Autodesk Inventor part; units mm, degrees
ref_plane "YZ Plane" through (0, 0, 0) normal (1, 0, 0) x (0, 1, 0)
ref_plane "XZ Plane" through (0, 0, 0) normal (0, 1, 0) x (-1, 0, 0)
ref_plane "XY Plane" through (0, 0, 0) normal (0, 0, 1) x (1, 0, 0)
sketch "Skizze1" plane through (0, 0, 0) normal (0, 0, 1) x (1, 0, 0)
  circle A0 centre (-60.768, 178.1277) radius 7
  circle A1 centre (-40.718, 169.3777) radius 1.6
  circle A2 centre (-40.718, 186.8777) radius 1.6
  line L0 (-23.718, 156.1277) -> (-23.718, 166.1277)
  arc A3 (-23.718, 166.1277) -> (-28.718, 171.1277) centre (-28.718, 166.1277) ccw
  line L1 (-28.718, 171.1277) -> (-29.418, 171.1277)
  arc A4 (-29.418, 185.1277) -> (-29.418, 171.1277) centre (-29.418, 178.1277) ccw
  line L2 (-40.918, 197.1277) -> (-40.918, 200.6277)
  line L3 (-40.918, 200.6277) -> (-60.918, 200.6277)
  line L4 (-68.918, 197.1277) -> (-76.918, 197.1277)
  line L5 (-76.918, 197.1277) -> (-76.918, 159.1277)
  line L6 (-76.918, 159.1277) -> (-68.918, 159.1277)
  line L7 (-64.918, 159.1277) -> (-26.718, 159.1277)
  line L8 (-26.718, 159.1277) -> (-26.718, 156.1277)
  line L9 (-26.718, 156.1277) -> (-23.718, 156.1277)
  line L10 (-36.5327, 178.1277) -> (-67.768, 178.1277) construction
  line L11 (-40.718, 169.3777) -> (-40.718, 186.8777) construction
  line L12 (-32.918, 197.1277) -> (-32.918, 193.6277)
  line L13 (-32.918, 193.6277) -> (-31.418, 193.6277)
  line L14 (-31.418, 193.6277) -> (-31.418, 190.1277)
  line L15 (-31.418, 190.1277) -> (-32.918, 190.1277)
  line L16 (-32.918, 190.1277) -> (-32.918, 188.6277)
  line L17 (-32.918, 188.6277) -> (-36.918, 188.6277)
  line L18 (-36.918, 188.6277) -> (-36.918, 190.1277)
  line L19 (-36.918, 190.1277) -> (-38.418, 190.1277)
  line L20 (-38.418, 190.1277) -> (-38.418, 193.6277)
  line L21 (-38.418, 193.6277) -> (-36.918, 193.6277)
  line L22 (-36.918, 197.1277) -> (-36.918, 193.6277)
  line L23 (-34.918, 197.9429) -> (-34.918, 190.1833) construction
  line L24 (-32.918, 197.1277) -> (-24.918, 197.1277)
  line L25 (-50.918, 190.3199) -> (-50.918, 199.5586) construction
  line L26 (-68.918, 190.1277) -> (-68.918, 188.6277)
  line L27 (-66.918, 197.9429) -> (-66.918, 190.1833) construction
  line L28 (-64.918, 197.1277) -> (-64.918, 193.6277)
  line L29 (-68.918, 188.6277) -> (-64.918, 188.6277)
  line L30 (-63.418, 193.6277) -> (-64.918, 193.6277)
  line L31 (-63.418, 190.1277) -> (-63.418, 193.6277)
  line L32 (-64.918, 188.6277) -> (-64.918, 190.1277)
  line L33 (-64.918, 190.1277) -> (-63.418, 190.1277)
  line L34 (-70.418, 190.1277) -> (-68.918, 190.1277)
  line L35 (-68.918, 193.6277) -> (-70.418, 193.6277)
  line L36 (-70.418, 193.6277) -> (-70.418, 190.1277)
  line L37 (-68.918, 197.1277) -> (-68.918, 193.6277)
  line L38 (-29.418, 185.1277) -> (-24.918, 185.1277)
  line L39 (-24.918, 185.1277) -> (-24.918, 197.1277)
  line L40 (-60.918, 200.6277) -> (-60.918, 197.1277)
  line L41 (-36.918, 197.1277) -> (-40.918, 197.1277)
  line L42 (-60.918, 197.1277) -> (-64.918, 197.1277)
  line L43 (-68.918, 162.6277) -> (-70.418, 162.6277)
  line L44 (-70.418, 162.6277) -> (-70.418, 166.1277)
  line L45 (-70.418, 166.1277) -> (-68.918, 166.1277)
  line L46 (-68.918, 166.1277) -> (-68.918, 167.6277)
  line L47 (-68.918, 167.6277) -> (-64.918, 167.6277)
  line L48 (-64.918, 167.6277) -> (-64.918, 166.1277)
  line L49 (-64.918, 166.1277) -> (-63.418, 166.1277)
  line L50 (-63.418, 166.1277) -> (-63.418, 162.6277)
  line L51 (-63.418, 162.6277) -> (-64.918, 162.6277)
  line L52 (-64.918, 159.1277) -> (-64.918, 162.6277)
  line L53 (-68.918, 159.1277) -> (-68.918, 162.6277)
  circle A5 centre (-49.518, 178.1277) radius 1.95
  point P0 (0, 0)
  point P1 (-56.218, 159.1277)
  point P2 (-36.918, 159.1277)
  point P3 (-40.718, 178.1277)
  dimension "d51" = 14
  dimension "d4" = 14
  dimension "d5" = 3
  dimension "d7" = 5
  dimension "d8" = 7
  dimension "d9" = 4.3
  dimension "d27" = 32
  dimension "d28" = 10
  dimension "d31" = 10
  dimension "d33" = 20
  dimension "d34" = 3.5
  dimension "d37" = 4
  dimension "d38" = 7
  dimension "d39" = 3.5
  dimension "d40" = 3.5
  dimension "d41" = 1.5
  dimension "d42" = 5.8
  dimension "d43" = 22.5
  dimension "d45" = 3
  dimension "d49" = 11.25
  dimension "d50" = 3.9
extrude "Extrusion1" add sketch "Skizze1" along normal mid plane 4 contours L9 L8 L7 L52 L51 L50 L49 L48 L47 L46 L45 L44 L43 L53 L6 L5 L4 L37 L35 L36 L34 L26 L29 L32 L33 L31 L30 L28 L42 L40 L3 L2 L41 L22 L21 L20 L19 L18 L17 L16 L15 L14 L13 L12 L24 L39 L38 A4 L1 A3 L0 | A5
sketch "Skizze2" plane through (0, 0, -2) normal (0, 0, -1) x (-1, 0, 0)
  circle A0 centre (60.768, 178.1277) radius 7
  circle A1 centre (40.718, 186.8777) radius 1.6
  circle A2 centre (40.718, 169.3777) radius 1.6
  line L0 (23.718, 166.1277) -> (23.718, 156.1277)
  line L1 (23.718, 156.1277) -> (26.718, 156.1277)
  line L2 (26.718, 156.1277) -> (26.718, 159.1277)
  line L3 (26.718, 159.1277) -> (64.918, 159.1277)
  line L4 (64.918, 159.1277) -> (64.918, 162.6277)
  line L5 (64.918, 162.6277) -> (63.418, 162.6277)
  line L6 (63.418, 162.6277) -> (63.418, 166.1277)
  line L7 (63.418, 166.1277) -> (64.918, 166.1277)
  line L8 (64.918, 166.1277) -> (64.918, 167.6277)
  line L9 (64.918, 167.6277) -> (68.918, 167.6277)
  line L10 (68.918, 167.6277) -> (68.918, 166.1277)
  line L11 (68.918, 166.1277) -> (70.418, 166.1277)
  line L12 (70.418, 166.1277) -> (70.418, 162.6277)
  line L13 (70.418, 162.6277) -> (68.918, 162.6277)
  line L14 (68.918, 162.6277) -> (68.918, 159.1277)
  line L15 (68.918, 159.1277) -> (76.918, 159.1277)
  line L16 (76.918, 159.1277) -> (76.918, 197.1277)
  line L17 (76.918, 197.1277) -> (68.918, 197.1277)
  line L18 (68.918, 197.1277) -> (68.918, 193.6277)
  line L19 (68.918, 193.6277) -> (70.418, 193.6277)
  line L20 (70.418, 193.6277) -> (70.418, 190.1277)
  line L21 (70.418, 190.1277) -> (68.918, 190.1277)
  line L22 (68.918, 190.1277) -> (68.918, 188.6277)
  line L23 (68.918, 188.6277) -> (64.918, 188.6277)
  line L24 (64.918, 188.6277) -> (64.918, 190.1277)
  line L25 (64.918, 190.1277) -> (63.418, 190.1277)
  line L26 (63.418, 190.1277) -> (63.418, 193.6277)
  line L27 (63.418, 193.6277) -> (64.918, 193.6277)
  line L28 (64.918, 193.6277) -> (64.918, 197.1277)
  line L29 (64.918, 197.1277) -> (60.918, 197.1277)
  line L30 (60.918, 197.1277) -> (60.918, 200.6277)
  line L31 (60.918, 200.6277) -> (40.918, 200.6277)
  line L32 (40.918, 200.6277) -> (40.918, 197.1277)
  line L33 (40.918, 197.1277) -> (36.918, 197.1277)
  line L34 (36.918, 197.1277) -> (36.918, 193.6277)
  line L35 (36.918, 193.6277) -> (38.418, 193.6277)
  line L36 (38.418, 193.6277) -> (38.418, 190.1277)
  line L37 (38.418, 190.1277) -> (36.918, 190.1277)
  line L38 (36.918, 190.1277) -> (36.918, 188.6277)
  line L39 (36.918, 188.6277) -> (32.918, 188.6277)
  line L40 (32.918, 188.6277) -> (32.918, 190.1277)
  line L41 (32.918, 190.1277) -> (31.418, 190.1277)
  line L42 (31.418, 190.1277) -> (31.418, 193.6277)
  line L43 (31.418, 193.6277) -> (32.918, 193.6277)
  line L44 (32.918, 193.6277) -> (32.918, 197.1277)
  line L45 (32.918, 197.1277) -> (24.918, 197.1277)
  line L46 (24.918, 197.1277) -> (24.918, 185.1277)
  line L47 (24.918, 185.1277) -> (29.418, 185.1277)
  arc A3 (29.418, 171.1277) -> (29.418, 185.1277) centre (29.418, 178.1277) ccw
  line L48 (29.418, 171.1277) -> (28.718, 171.1277)
  arc A4 (28.718, 171.1277) -> (23.718, 166.1277) centre (28.718, 166.1277) ccw
  circle A5 centre (40.718, 169.3777) radius 1.6
  line L49 (42.9634, 171.623) -> (43.7853, 168.5558)
  line L50 (43.7853, 168.5558) -> (41.5399, 166.3104)
  line L51 (41.5399, 166.3104) -> (38.4727, 167.1323)
  line L52 (38.4727, 167.1323) -> (37.6508, 170.1995)
  line L53 (37.6508, 170.1995) -> (39.8962, 172.4449)
  line L54 (39.8962, 172.4449) -> (42.9634, 171.623)
  line L55 (42.9634, 189.123) -> (43.7853, 186.0558)
  line L56 (43.7853, 186.0558) -> (41.5399, 183.8104)
  line L57 (41.5399, 183.8104) -> (38.4727, 184.6323)
  line L58 (38.4727, 184.6323) -> (37.6508, 187.6995)
  line L59 (37.6508, 187.6995) -> (39.8962, 189.9449)
  line L60 (39.8962, 189.9449) -> (42.9634, 189.123)
  line L61 (38.418, 190.1277) -> (36.918, 188.6277) construction
  point P0 (0, 0)
  dimension "d52" = 5.5
extrude "Extrusion2" cut sketch "Skizze2" against normal blind 2 contours L49 L50 L51 L52 L53 L54 | L55 L56 L57 L58 L59 L60
sketch "Skizze3" plane through (-64.918, 159.1277, 2) normal (0, -1, 0) x (1, 0, 0)
  line L0 (0, 0) -> (38.2, 0)
  line L1 (12, -4) -> (16, -4)
  line L2 (16, -4) -> (16, 0)
  line L3 (16, 0) -> (12, 0)
  line L4 (12, 0) -> (12, -4)
  line L5 (-12, -4) -> (-12, 0)
  point P0 (64.918, -2)
  point P1 (-2, -2)
  dimension "d55" = 4
  dimension "d57" = 24
extrude "Extrusion3" add sketch "Skizze3" along normal blind 2
properties part number "Motorhalter_links"
Build history of the part. All positions in model axes, mm. A direction names the side the tool comes from. Round coordinates to 2 decimals unless told otherwise and drop trailing zeros. Write each loop counter-clockwise with the first axis right and the second up, starting at its lowest first coordinate (ties: lowest second). Pieces come first, ordered by that corner, then holes. Notation, with made-up numbers: (25, 80) - (45, 80) arc R23 cw to (45, 106) - close; hole circle Ø11 at (69.25, -28.75). An arc over 180 degrees is marked (long way). One line per question, with ' | ' between items.
1. Mould opens along X. For faces 6 (the face through (-60.918, 199, 0)), 7 (the face through (-51, 179, -2)), 8 (the face through (-70.418, 192, 0)) say: released by +X, released by -X, zero draft, split by the parting line, or undercut.
Results are:
face 6: released by -X | face 7: zero draft | face 8: undercut
2. Band-saw the part on B-B, the plane y = 161.5. Write the cut outline in (x, z).
Results are:
outline: (-76.92, -2) - (-68.92, -2) - (-68.92, 2) - (-76.92, 2) - close; (-64.92, -2) - (-23.72, -2) - (-23.72, 2) - (-64.92, 2) - close
3. Band-saw the part on C-C, the plane x = -60. Write the cut outline in (y, z), and give its area (3 significant figures).
Results are:
outline: (159.13, -2) - (171.17, -2) - (171.17, 2) - (159.13, 2) - close; (185.09, -2) - (200.63, -2) - (200.63, 2) - (185.09, 2) - close | area: 110 mm^2
4. Tool access for faces 1 (the face through (-64.918, 195, 0)), 2 (the face through (-38.418, 192, 0)), 3 (the face through (-67, 167.628, 0)), 4 (the face through (-29, 197.128, 0)), 5 (the face through (-42.68, 184.95, -1.01)): list every direction of +Z, -Z, +X, -X, +Y, -Y with a clear straight run to the whole face (end or side of a thin tool).
Results are:
face 1: +Z, -Z, +Y | face 2: +Z, -Z | face 3: +Z, -Z, -Y | face 4: +Z, -Z, +X, +Y | face 5: -Z
5. Band-saw the part on A-A, the plane y = 196.5. Write the cut outline in (x, z), and give its area (3 significant figures).
Results are:
outline: (-76.92, -2) - (-68.92, -2) - (-68.92, 2) - (-76.92, 2) - close; (-64.92, -2) - (-36.92, -2) - (-36.92, 2) - (-64.92, 2) - close; (-32.92, -2) - (-24.92, -2) - (-24.92, 2) - (-32.92, 2) - close | area: 176 mm^2
6. Drop flat-ended pins along their axis: pin 1 Ø1 at (x, z) = (-62, -1) entering from +Y; pin 2 Ø1.2 at (x, z) = (-66.5, 0.5) entering from -Y; pin 3 Ø1.2 at (y, z) = (191, 0.5) entering from +X. Give the stop position or say it passes through.
Results are:
pin 1: y = 197.13 | pin 2: y = 167.63 | pin 3: x = -24.92
7. Band-saw the part on D-D, the plane x = -73. Write the cut outline in (y, z).
Results are:
outline: (159.13, -2) - (197.13, -2) - (197.13, 2) - (159.13, 2) - close
8. Drill centre lines: line 1 along X through (y, z) = (189.5, 0.8); line 2 along X through (y, z) = (192.5, -1.6); line 3 along X through (y, z) = (178, 0.45). Where is each one in solid material? Low to high. Write a range as from..to.
Results are:
line 1: -76.92..-68.92, -64.92..-36.92, -32.92..-24.92 | line 2: -76.92..-70.42, -63.42..-38.42, -31.42..-24.92 | line 3: -76.92..-67.77, -53.77..-36.42
